Source: CAD feature listing. Evaluate the final solid. Frame: model axes, mm. Face numbers are marked on the shaded views. A direction names the side the tool comes from. Round coordinates to 2 decimals unless told otherwise and drop trailing zeros. Write each loop counter-clockwise with the first axis right and the second up, starting at its lowest first coordinate (ties: lowest second). Pieces come first, ordered by that corner, then holes. Notation, with made-up numbers: (48.25, 73.25) -> (69.25, 73.25) arc R18 cw to (69.25, 86.25) -> close; hole circle Ø9 at (86, 66.5). An arc over 180 degrees is marked (long way). Put each result on its own line as item: value.
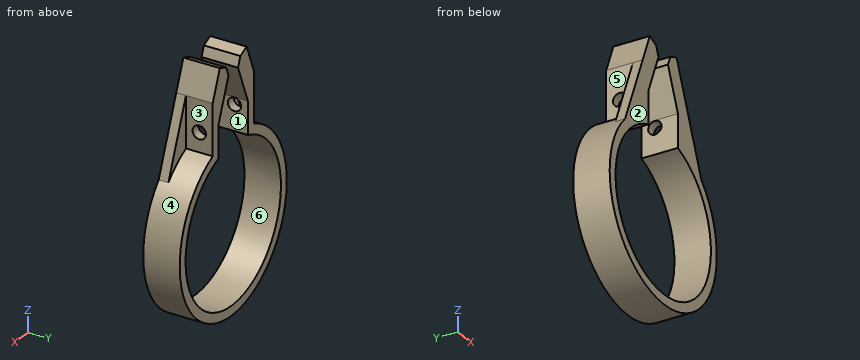
```python
from build123d import *

# Parameters (mm, degrees)
BOSS_EXTRUDE1_DEPTH = 15
BOSS_EXTRUDE2_DEPTH = 4
CUT_EXTRUDE1_DEPTH  = 4
BOSS_EXTRUDE3_DEPTH = 15
CHAMFER1_SIZE       = 3
SKETCH6_R           = 2.75
CUT_EXTRUDE2_DEPTH  = 50


with BuildPart() as part:
    # Sketch1 → Boss-Extrude1 (new body)
    with BuildSketch(Plane(origin=(0, 0, 0), x_dir=(1, 0, 0), z_dir=(0, 1, 0))):
        with BuildLine():
            Line((-14, -33.708307581), (-14, -55))
            Line((-14, -55), (-10, -55))
            Line((-10, -55), (-10, -30.923292192))
            ThreePointArc((-10, -30.923292192), (0, 32.5), (10, -30.923292192))
            Line((10, -30.923292192), (10, -55))
            Line((10, -55), (14, -55))
            Line((14, -55), (14, -33.708307581))
            ThreePointArc((14, -33.708307581), (0, 36.5), (-14, -33.708307581))
        make_face()
    extrude(amount=BOSS_EXTRUDE1_DEPTH)

    # Sketch2 → Boss-Extrude2 (add)
    with BuildSketch(Plane.XZ):
        Polygon((-26, 22.856938123), (-14, 33.708307581), (-14, 55), (-26, 55), align=None)
        Polygon((14, 55), (26, 55), (26, 22.856938123), (14, 33.708307581), align=None)
    extrude(amount=-BOSS_EXTRUDE2_DEPTH)

    # Sketch4 → Cut-Extrude1 (cut)
    with BuildSketch(Plane(origin=(0, 4, 0), x_dir=(1, 0, 0), z_dir=(0, 1, 0))):
        Polygon((-26, -25.617376915), (-14, -55), (-32.323218547, -64.259569624), align=None)
        Polygon((14, -55), (26, -25.617376915), (31.225077356, -59.629784812), align=None)
    extrude(amount=-CUT_EXTRUDE1_DEPTH, mode=Mode.SUBTRACT)

    # Sketch5 → Boss-Extrude3 (add)
    with BuildSketch(Plane.XZ):
        Polygon((-9.146083297, 66.885067081), (-14, 55), (-10, 55), (-10, 44.654426435), (-2.09670025, 64.00606624), align=None)
        Polygon((10, 55), (14, 55), (9.146083297, 66.885067081), (2.09670025, 64.00606624), (10, 44.654426435), align=None)
    extrude(amount=-BOSS_EXTRUDE3_DEPTH)

    # Chamfer1
    chamfer1_edges = [part.edges().sort_by_distance(p)[0] for p in [
        (-2.09670025, 7.5, 64.00606624),
        (2.09670025, 7.5, 64.00606624),
    ]]
    chamfer(chamfer1_edges, length=CHAMFER1_SIZE)

    # Sketch6 → Cut-Extrude2 (cut)
    with BuildSketch(Plane(origin=(14, 0, 0), x_dir=(0, 0, -1), z_dir=(1, 0, 0))):
        with Locations((-41.708307581, 9.466509398)):
            Circle(SKETCH6_R)
    extrude(amount=-CUT_EXTRUDE2_DEPTH, mode=Mode.SUBTRACT)


solid = part.part
```
Q1. Cut plane D-D on x = 18.5. Output: boundary loops of the cut face in (y, z).
Ans:
outline: (0, -31.46) -> (15, -31.46) -> (15, -26.72) -> (0, -26.72) -> close; (0, 26.72) -> (15, 26.72) -> (15, 31.46) -> (4, 31.46) -> (4, 43.98) -> (0, 43.98) -> close
Q2. Reachability of the marked faces 1, 2 and 3 from +Z, -Z, +X, -X, +Y, -Y: full face, straight path, thin tool, end or side. Return the list, or none.
Ans:
face 1: +Y, -Y
face 2: +Z, -Z, +X, -X, -Y
face 3: +Z, +X, +Y
Q3. Draft query along Z for the marked faces 4, 5 and 6. Return one class per face: +Z half, -Z half, draft (parallel to the pull), parting line (faces both ways), or undercut.
Ans:
face 4: parting line
face 5: draft
face 6: undercut
Q4. Cut plane B-B on x = -19. Output: boundary loops of the cut face in (y, z).
Ans:
outline: (0, -31.16) -> (15, -31.16) -> (15, -26.37) -> (0, -26.37) -> close; (0, 26.37) -> (15, 26.37) -> (15, 31.16) -> (4, 31.16) -> (4, 42.76) -> (0, 42.76) -> close
Q5. Pin query (flat end, axial travel): pin 1 (6 mm diameter, centred on x = 18.5, z = 21.5, fed in from +Y); pin 2 (3 mm diameter, centred on y = 9, z = -23, fed in from +X); pin 3 (1.5 mm diameter, centred on x = 5, y = 4, fed in from -Z); pin 4 (3.5 mm diameter, centred on y = 11.5, z = 41.5, fed in from +X). Return the tip coordinate at first contact, or that it passes through.
Ans:
pin 1: passes through
pin 2: stops at x = 29.5
pin 3: stops at z = -36.25
pin 4: stops at x = 14
Q6. Cut plane C-C on z = 48. Output: boundary loops of the cut face in (x, y).
Ans:
outline: (-16.86, 0) -> (-8.63, 0) -> (-8.63, 15) -> (-14, 15) -> (-14, 4) -> (-16.86, 4) -> close; (8.63, 0) -> (16.86, 0) -> (16.86, 4) -> (14, 4) -> (14, 15) -> (8.63, 15) -> close
Q7. Cut plane A-A on z = 0. Output: boundary loops of the cut face in (x, y), and give its area (3 significant figures).
Ans:
outline: (-36.5, 0) -> (-32.5, 0) -> (-32.5, 15) -> (-36.5, 15) -> close; (32.5, 0) -> (36.5, 0) -> (36.5, 15) -> (32.5, 15) -> close
area: 120 mm^2
Q8. Material intervals for line 1 (Z direction, x = -1, y = 5.25); line 2 (X direction, y = 6.5, z = 61); line 3 (X direction, y = 3.25, z = 44), sorted ascending. Write a range as [from, to].
Ans:
line 1: z = [-36.49, -32.48]
line 2: x = [-11.55, -3.32], [3.32, 11.55]
line 3: x = [-18.49, -10], [10, 18.49]
